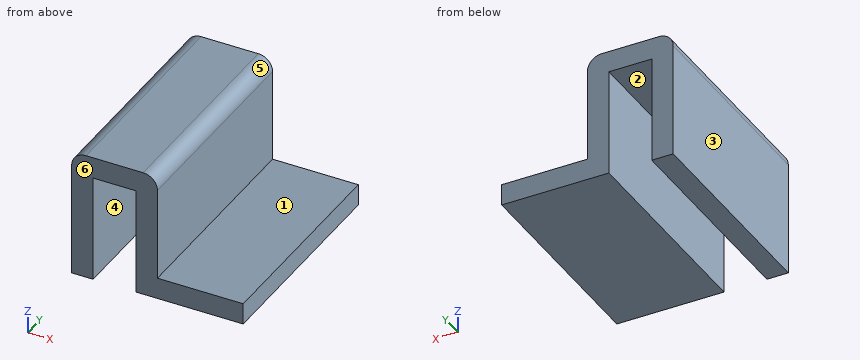
```python
from build123d import *

# Parameters (mm, degrees)
F1_DEPTH = 30
F2_R     = 2
F3_R     = 2


with BuildPart() as f1:
    # F0 (on Front) → F1 (new body)
    with BuildSketch(Plane.XZ):
        Polygon((-6, 0), (-6, 15), (0, 15), (0, 0), (15, 0), (15, 3), (3, 3), (3, 18), (-9, 18), (-9, 0), align=None)
    extrude(amount=F1_DEPTH)

    # F2
    f2_edges = [f1.edges().sort_by_distance(p)[0] for p in [
        (3, -15, 18),
    ]]
    fillet(f2_edges, radius=F2_R)

    # F3
    f3_edges = [f1.edges().sort_by_distance(p)[0] for p in [
        (-9, -15, 18),
    ]]
    fillet(f3_edges, radius=F3_R)


solid = f1.part
```
The listing builds one solid part. Answer for the finished solid, in the listing's coordinates (mm). Face numbers are marked on the shaded views. A direction names the side the tool comes from. Round coordinates to 2 decimals unless told otherwise and drop trailing zeros. Loops run counter-clockwise (first coordinate to the right, second up) from the corner with the lowest first, then second, coordinate; pieces in that order, holes last.
Q1. Section D-D, the plane x = -1.25 is taken. Determine the outline of the cut face in (y, z), then the cut area to 3 significant figures.
Q2. Find the intervals of material crossed by line 1 (X direction, y = -0.75, z = 1.5); line 2 (X direction, y = -11, z = 8); line 3 (Z direction, x = -1.5, y = -3.75), in increasing order.
Q3. Section B-B, the plane y = -21.25 is taken. Determine the outline of the cut face in (x, z).
Q4. Which of the six approach directions +Z, -Z, +X, -X, +Y, -Y give full straight-line access (tool end or side, diameter ignored) to the marked faces 1, 2 and 3?
Q5. Section C-C, the plane z = 1.5 is taken. Determine the outline of the cut face in (x, y), then the cut area to 3 significant figures.
Q6. Section A-A, the plane z = 5.25 is taken. Determine the outline of the cut face in (x, y), then the cut area to 3 significant figures.
Q7. For a pull along X with two mould halves and no side action, classify the marked faces 4, 5 and 6 as released by +X, released by -X, zero draft, split by the parting line, or undercut.
Q8. Given pin 1 Ø13 at (x, y) = (8, -10) entering from +Z; pin 2 Ø5 at (x, z) = (5, 6.5) entering from +Y; pin 3 Ø4 at (y, z) = (-13, 7.5) entering from +X; pin 4 Ø1.5 at (x, y) = (-4.5, -4.5) entering from -Z, each flat-ended and moving along its own axis, determine where each tip first touches the part or whether it passes through.
Completed:
1. outline: (-30, 15) - (0, 15) - (0, 18) - (-30, 18) - close
1. area: 90.0 mm2
2. line 1: x = -9 to -6, 0 to 15
2. line 2: x = -9 to -6, 0 to 3
2. line 3: z = 15 to 18
3. outline: (-9, 0) - (-6, 0) - (-6, 15) - (0, 15) - (0, 0) - (15, 0) - (15, 3) - (3, 3) - (3, 16) arc R2 ccw to (1, 18) - (-7, 18) arc R2 ccw to (-9, 16) - close
4. face 1: +Z, +X, +Y, -Y
4. face 2: -Z, +Y, -Y
4. face 3: +Z, -Z, -X, +Y, -Y
5. outline: (-9, -30) - (-6, -30) - (-6, 0) - (-9, 0) - close; (0, -30) - (15, -30) - (15, 0) - (0, 0) - close
5. area: 540 mm2
6. outline: (-9, -30) - (-6, -30) - (-6, 0) - (-9, 0) - close; (0, -30) - (3, -30) - (3, 0) - (0, 0) - close
6. area: 180 mm2
7. face 4: undercut
7. face 5: released by +X
7. face 6: zero draft
8. pin 1: stops at z = 17.94
8. pin 2: stops at y = 0
8. pin 3: stops at x = 3
8. pin 4: stops at z = 15
